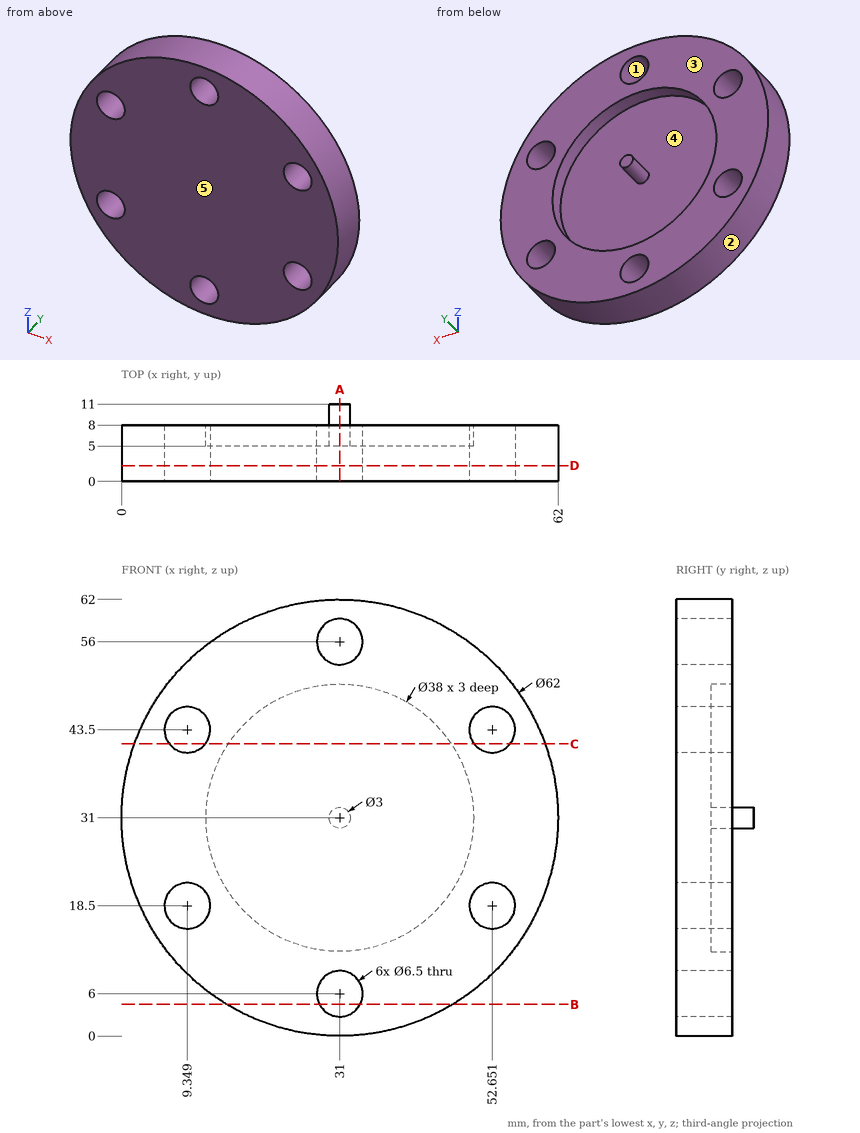
Here's the drawing with two shaded views (mm, measured from the low corner). I have some questions. A direction names the side the tool comes from. Coordinates: 2 decimals unless noted, no trailing zeros. Loops run counter-clockwise (first coordinate to the right, second up) from the corner with the lowest first, then second, coordinate; pieces in that order, holes last. Notation, with made-up numbers: M -18.5,25.25 L 34.5,25.25 A36 cw 34.5,64.25 Z; hole C 27,60 d6. An arc over 180 degrees is marked long. Answer as CSV lines item,"result". Start each with the question number.
1. Suppose I cut it at C-C, the plane z = 41.5. List the corners of the cut face in (x, y) for me (1 decimal), plus the area to 3 significant figures.
2. If I drill on probe 1 along Z at (x, y) = (31, 3.25); probe 2 along X at (y, z) = (6.5, 31); probe 3 along Z at (x, y) = (10.5, 4.75) (1 decimal), over which ranges is the centre line in solid material (lowest first)? Write a range as [from, to].
3. For the marked faces 4 and 5, which set-ups out of +Z, -Z, +X, -X, +Y, -Y let a thin tool reach every point of the face, with its end or its side?
4. Thinking about a two-plate mould opening in Z: for the marked faces 1, 2 and 3, which applies, +Z half, -Z half, draft (parallel to the pull), parting line (faces both ways), or undercut?
5. Suppose I cut it at A-A, the plane x = 31. List the corners of the cut face in (y, z) for me, plus the area to 3 significant figures.
6. Suppose I cut it at B-B, the plane z = 4.5. List the corners of the cut face in (x, y) for me (1 decimal).
7. Suppose I cut it at D-D, the plane y = 2.25. Count the separate pieces of the cut face and the enclosed holes in it, plus the area to 3 significant figures.
8. For pin 1 Ø4 at (x, y) = (30.5, 1.5) entering from -Z; pin 2 Ø10.5 at (x, z) = (9.35, 43.5) entering from -Y; pin 3 Ø6 at (x, z) = (31, 56) entering from +Y; pin 4 Ø5 at (y, z) = (5.5, 41.5) entering from +X, each with a flat end and sliding along its axis, tell me the tip position at first contact or that it passes through.
Output:
1,outline,"M 1.8,0 L 6.8,0 L 6.8,8 L 1.8,8 Z; M 11.9,0 L 50.1,0 L 50.1,8 L 46.8,8 L 46.8,5 L 15.2,5 L 15.2,8 L 11.9,8 Z; M 55.2,0 L 60.2,0 L 60.2,8 L 55.2,8 Z"
1,area,"290 mm^2"
2,probe 1,"z = [0, 2.75], [9.25, 52.75], [59.25, 62]"
2,probe 2,"x = [0, 12], [29.5, 32.5], [50, 62]"
2,probe 3,"z = [7.7, 15.5], [21.5, 40.5], [46.5, 54.3]"
3,face 4,"+Y"
3,face 5,"+Z, -Z, +X, -X, -Y"
4,face 1,"undercut"
4,face 2,"parting line"
4,face 3,"draft"
5,outline,"M 0,0 L 8,0 L 8,2.75 L 0,2.75 Z; M 0,9.25 L 8,9.25 L 8,12 L 5,12 L 5,29.5 L 11,29.5 L 11,32.5 L 5,32.5 L 5,50 L 8,50 L 8,52.75 L 0,52.75 Z; M 0,59.25 L 8,59.25 L 8,62 L 0,62 Z"
5,area,"296 mm^2"
6,outline,"M 14.9,0 L 28.1,0 L 28.1,8 L 14.9,8 Z; M 33.9,0 L 47.1,0 L 47.1,8 L 33.9,8 Z"
7,separate pieces,"1"
7,enclosed holes,"6"
7,area,"2,820 mm^2"
8,pin 1,"stops at z = 0"
8,pin 2,"stops at y = 0"
8,pin 3,"passes through"
8,pin 4,"stops at x = 60.95"
